Autodesk Inventor part; units mm, degrees
ref_plane "YZ Plane" through (0, 0, 0) normal (1, 0, 0) x (0, 1, 0)
ref_plane "XZ Plane" through (0, 0, 0) normal (0, 1, 0) x (-1, 0, 0)
ref_plane "XY Plane" through (0, 0, 0) normal (0, 0, 1) x (1, 0, 0)
sketch "Boceto1" plane through (0, 0, 0) normal (0, 0, 1) x (1, 0, 0)
  line L0 (-22.5, 22.5) -> (22.5, 22.5)
  line L1 (22.5, 22.5) -> (22.5, -22.5)
  line L2 (22.5, -22.5) -> (-22.5, -22.5)
  line L3 (-22.5, -22.5) -> (-22.5, 22.5)
  line L4 (-20, 17.5) -> (20, 17.5)
  line L5 (20, 17.5) -> (20, -17.5)
  line L6 (20, -17.5) -> (-20, -17.5)
  line L7 (-20, -17.5) -> (-20, 17.5)
  point P0 (0, 0)
  point P1 (-22.5, 0)
  point P2 (0, 22.5)
  point P3 (-20, 0)
  point P4 (0, 17.5)
  dimension "d0" = 45
  dimension "d1" = 45
  dimension "d2" = 35
  dimension "d3" = 40
extrude "Extrusión1" add sketch "Boceto1" against normal blind 2.5 contours L0 L1 L2 L3 | L4 L5 L6 L7
extrude "Extrusión2" add sketch "Boceto1" along normal blind 5 contours L4 L5 L6 L7
equation "\"d1\" = d0"
properties part number "pantalla"
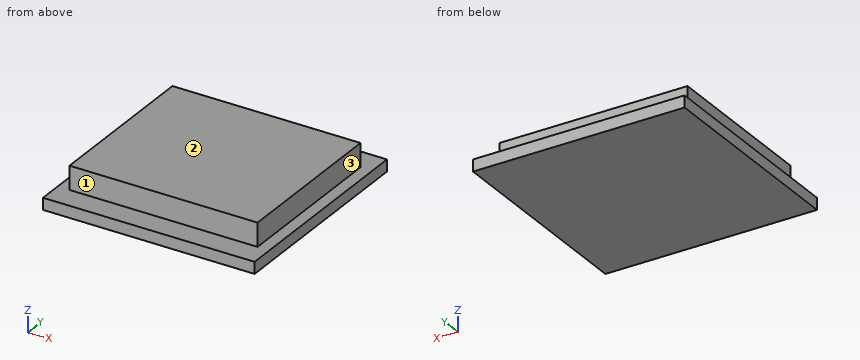
Can you work these out from the model? Positions are in its coordinate system, mm. Face numbers are marked on the shaded views. A direction names the side the tool comes from. Coordinates: 2 decimals unless noted, no trailing zeros. Loops run counter-clockwise (first coordinate to the right, second up) from the corner with the lowest first, then second, coordinate; pieces in that order, holes last. Notation, with made-up numbers: M -36,12 L -28,12 A27 ccw -28,48 Z; hole C -25.5,78.5 d1. An arc over 180 degrees is marked long. Return JSON: item names as keys, results as strings. Group by question number.
Item 1: On a 3-axis mill with a long thin cutter (end or side, diameter ignored), from which of +Z, -Z, +X, -X, +Y, -Y can I reach the whole of each face in a straight line? I mean the marked faces 1, 2 and 3. Say none if no direction works.
Item 2: Imagine slicing it at C-C (z = 1.75). Please give me the cut outline in (x, y).
Item 3: I'm going to push flat-ended pins straight in: pin 1 Ø2.5 at (x, z) = (-0.5, 3) entering from -Y; pin 2 Ø1.5 at (y, z) = (-8, 3) entering from -X; pin 3 Ø1.5 at (x, z) = (7.5, 3.5) entering from +Y; pin 4 Ø1.5 at (x, z) = (-14, 0.5) entering from -Y. Where does each tip first touch, or does it pass through?
Item 4: Imagine slicing it at A-A (x = -8). Please give me the cut outline in (y, z), and give its area (4 significant figures).
Item 5: If I drill on L1, parallel to Y at x = -2, z = 4.5; L2, parallel to Z at x = 17, y = -19.5; L3, parallel to X at y = 11, z = 3.5, over which ranges is the centre line in solid material (lowest first)? Write a range as from..to.
Item 6: Imagine slicing it at B-B (y = 6). Please give me the cut outline in (x, z), and give its area (4 significant figures).
Verdict:
{
 "1": {"face 1": "+Z, +X, -X, -Y", "face 2": "+Z, +X, -X, +Y, -Y", "face 3": "+Z, +X, +Y, -Y"},
 "2": {"outline": "M -20,-17.5 L 20,-17.5 L 20,17.5 L -20,17.5 Z"},
 "3": {"pin 1": "stops at y = -17.5", "pin 2": "stops at x = -20", "pin 3": "stops at y = 17.5", "pin 4": "stops at y = -22.5"},
 "4": {"outline": "M -22.5,-2.5 L 22.5,-2.5 L 22.5,0 L 17.5,0 L 17.5,5 L -17.5,5 L -17.5,0 L -22.5,0 Z", "area": "287.5 mm^2"},
 "5": {"L1": "y = -17.5..17.5", "L2": "z = -2.5..0", "L3": "x = -20..20"},
 "6": {"outline": "M -22.5,-2.5 L 22.5,-2.5 L 22.5,0 L 20,0 L 20,5 L -20,5 L -20,0 L -22.5,0 Z", "area": "312.5 mm^2"}
}
